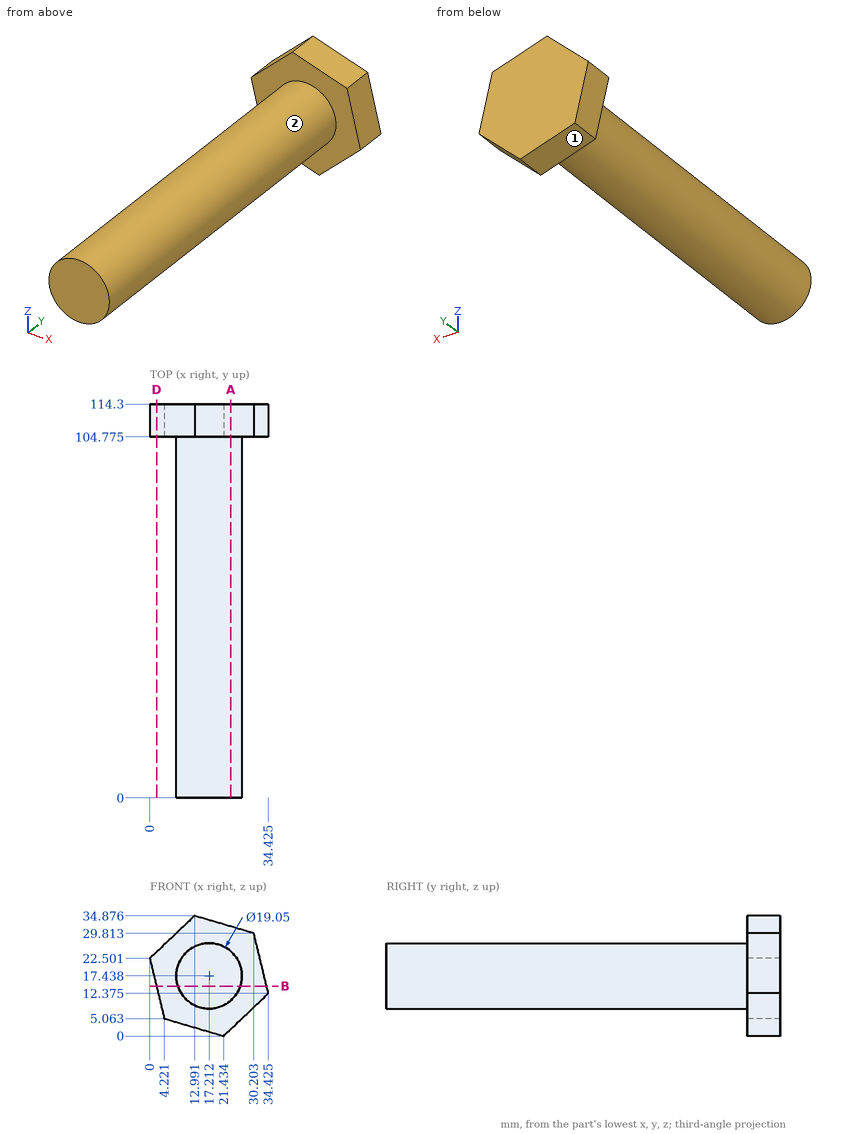
Verification items for this drawing (mm, ordinates from the low corner). A direction names the side the tool comes from. Coordinates: 2 decimals unless noted, no trailing zeros. Write each loop counter-clockwise with the first axis right and the second up, starting at its lowest first coordinate (ties: lowest second). Pieces come first, ordered by that corner, then holes. Notation, with made-up numbers: (6, -28) - (65, -28) arc R10 ccw to (65, -19) - close; hole circle Ø7 at (-16, 81). An arc over 180 degrees is marked (long way). One line per question, with ' | ' between items.
Item 1: Gauge pin test, flat ends, axial feed: P1, Ø1.5, axis at y = 37.5, z = 21.5, coming from the -X side; P2, Ø1.5, axis at x = 10, z = 7.5, coming from the -Y side (3 decimals); P3, Ø12, axis at x = 22, y = 60, coming from the -Z side. Record the tip position at first contact, or that the pin passes through.
Determined:
P1: stops at x = 8.28 | P2: stops at y = 104.775 | P3: stops at z = 7.91
Item 2: Sectioned sample at A-A on x = 23.5. Record the boundary of the cut face in (y, z) (1 decimal).
Determined:
outline: (0, 10.3) - (104.8, 10.3) - (104.8, 2) - (114.3, 2) - (114.3, 31.8) - (104.8, 31.8) - (104.8, 24.6) - (0, 24.6) - close
Item 3: Sectioned sample at D-D on x = 2. Record the boundary of the cut face in (y, z) (1 decimal).
Determined:
outline: (104.8, 14.2) - (114.3, 14.2) - (114.3, 24.4) - (104.8, 24.4) - close
Item 4: Sectioned sample at B-B on z = 14.5. Record the boundary of the cut face in (x, y) (1 decimal), plus the area to 3 significant figures.
Determined:
outline: (1.9, 104.8) - (8.2, 104.8) - (8.2, 0) - (26.3, 0) - (26.3, 104.8) - (33.9, 104.8) - (33.9, 114.3) - (1.9, 114.3) - close | area: 2,200 mm2
Item 5: Access from +Z, -Z, +X, -X, +Y, -Y to the whole of each face (thin tool, end or side, straight path). Record for the marked faces 1 and 2.
Determined:
face 1: -Z, -X, +Y, -Y | face 2: -Y
Item 6: Thickness scan on line 1 (Y direction, x = 31, z = 16) (1 decimal); line 2 (X direction, y = 38.5, z = 21) (1 decimal); line 3 (X direction, y = 53.5, z = 11). Record the ranges inside material, lowest first. Write a range as [from, to].
Determined:
line 1: y = [104.8, 114.3] | line 2: x = [8.4, 26] | line 3: x = [10.19, 24.23]
